from build123d import *

# Parameters (mm, degrees)
SKETCH1_R          = 10
EXTRUDE1_DEPTH     = 8
EXTRUDE2_START     = 1
SKETCH3_R          = 10
SKETCH3_R_2        = 9
EXTRUDE2_DEPTH     = 1
SKETCH2_R          = 6.3
CUT_EXTRUDE1_DEPTH = 17.763054614


with BuildPart() as part:
    # Sketch1 → Extrude1 (new body)
    with BuildSketch(Plane.XY):
        Circle(SKETCH1_R)
    extrude(amount=EXTRUDE1_DEPTH)

    # Sketch3 → Extrude2 (add)
    with BuildSketch(Plane(origin=(0, 0, 0), x_dir=(-1, 0, 0), z_dir=(0, 0, -1)).offset(EXTRUDE2_START)):
        Circle(SKETCH3_R)
        Circle(SKETCH3_R_2, mode=Mode.SUBTRACT)
    extrude(amount=-EXTRUDE2_DEPTH)

    # Sketch2 → Cut-Extrude1 (cut, through all)
    with BuildSketch(Plane.XY.offset(8)):
        Circle(SKETCH2_R)
    extrude(amount=-CUT_EXTRUDE1_DEPTH, mode=Mode.SUBTRACT)


solid = part.part
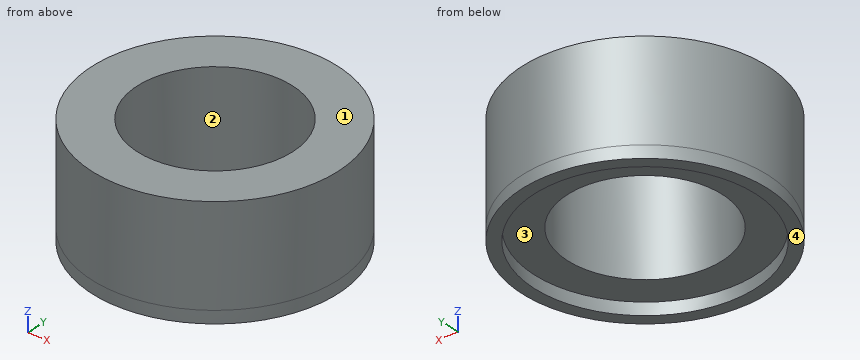
Source: CAD feature listing. Evaluate the final solid. Frame: model axes, mm. Face numbers are marked on the shaded views. A direction names the side the tool comes from. Round coordinates to 2 decimals unless told otherwise and drop trailing zeros. Loops run counter-clockwise (first coordinate to the right, second up) from the corner with the lowest first, then second, coordinate; pieces in that order, holes last. Notation, with made-up numbers: (48.25, 16) -> (61.25, 16) arc R11 cw to (61.25, 33) -> close; hole circle Ø8 at (59, 80). An arc over 180 degrees is marked (long way). Answer as a JSON object with one key per item and string values. Group by question number.
Q1. Section query A-A (x = 0). Output: boundary loops of the cut face in (y, z).
Q2. Access query for the marked faces 3 and 4. Directions: +Z, -Z, +X, -X, +Y, -Y. A direction counts if a zero-diameter tool reaches every point of the face in a straight line with its end or side. Return the directions, or none.
Q3. Contact query for flat-ended pins moving along their axis: P1, Ø4, axis at y = -5.5, z = 4.5, coming from the +X side; P2, Ø2, axis at y = 6.5, z = 0.5, coming from the -X side; P3, Ø9, axis at x = 3.5, y = -2.5, coming from the -Z side. Output: stop coordinate, or through.
Q4. Mould query, pull axis X, two halves, no side actions, for the marked faces 1 and 2. Classes: pulls with the +X half, pulls with the -X half, needs draft (parallel to the pull), parting line crosses it, or undercut.
Q5. Ray query, line 1 (Y direction, x = 0, z = 4.75); line 2 (Y direction, x = 0, z = -0.5); line 3 (Z direction, x = 8, y = -3.5). Return the intervals inside material, ascending. Write a range as from..to.
Q6. Section query D-D (x = -7.25). Output: boundary loops of the cut face in (y, z).
Q7. Section query C-C (z = 5.5). Output: boundary loops of the cut face in (x, y).
Completed:
{
 "1": {"outline": "(-10, -1) -> (-9, -1) -> (-9, 0) -> (-6.3, 0) -> (-6.3, 8) -> (-10, 8) -> close; (6.3, 0) -> (9, 0) -> (9, -1) -> (10, -1) -> (10, 8) -> (6.3, 8) -> close"},
 "2": {"face 3": "-Z", "face 4": "-Z, +X, -X, +Y, -Y"},
 "3": {"P1": "x = 9.37", "P2": "x = -8.35", "P3": "z = 0"},
 "4": {"face 1": "needs draft", "face 2": "undercut"},
 "5": {"line 1": "-10..-6.3, 6.3..10", "line 2": "-10..-9, 9..10", "line 3": "0..8"},
 "6": {"outline": "(-6.89, -1) -> (-5.33, -1) -> (-5.33, 0) -> (5.33, 0) -> (5.33, -1) -> (6.89, -1) -> (6.89, 8) -> (-6.89, 8) -> close"},
 "7": {"outline": "circle Ø20 at (0, 0); hole circle Ø12.6 at (0, 0)"}
}
